Design review of the part shown in the three views and the two pictorial views. Dimensions are in mm from the part's minimum x, y and z. A direction names the side the tool comes from. Give positions to 0.01 mm unless a question says otherwise; leave off trailing zeros. Write each loop counter-clockwise with the first axis right and the second up, starting at its lowest first coordinate (ties: lowest second). Pieces come first, ordered by that corner, then holes. Notation, with made-up numbers: (58, -27.5) -> (90, -27.5) arc R19 cw to (90, 1.5) -> close; hole circle Ø3 at (6, 56). An arc over 180 degrees is marked (long way). Use CSV: the item, a comma, the result in double quotes.
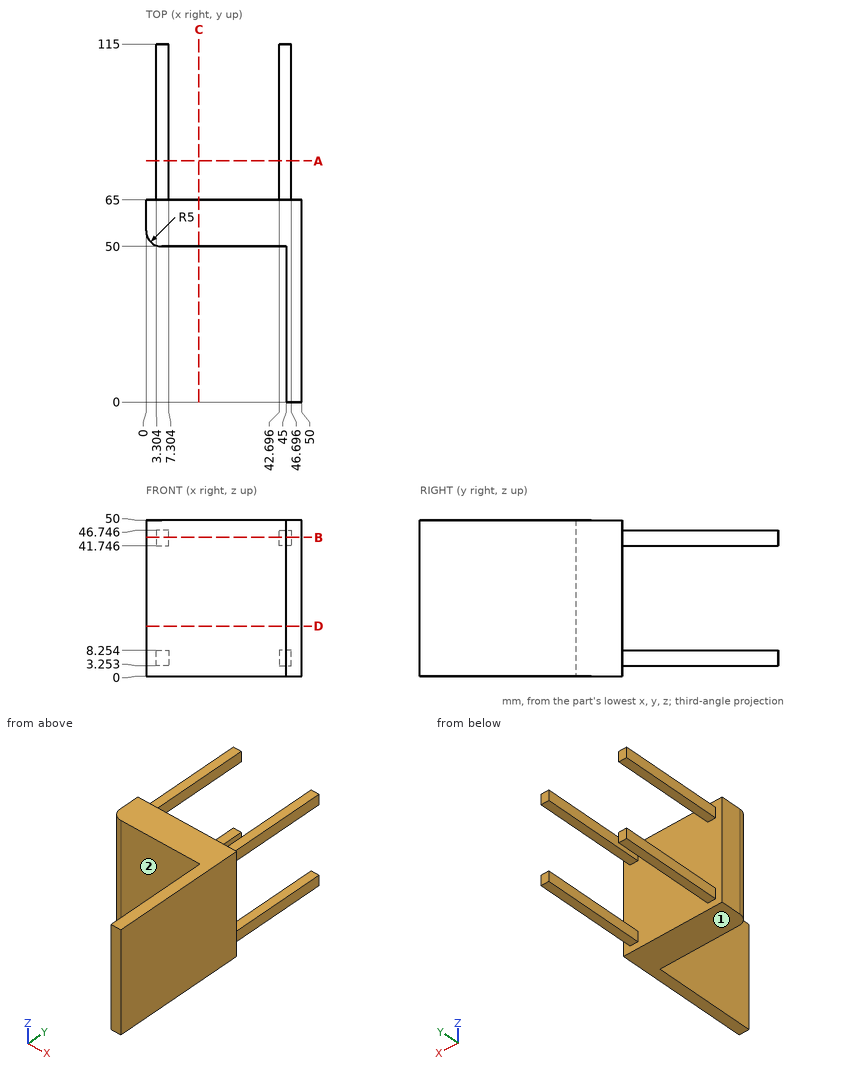
Q1. Consider section B-B (z = 44.5). Write out the cut boundary in (x, y) (1 decimal).
Derived:
outline,"(0, 55) arc R5 ccw to (5, 50) -> (45, 50) -> (45, 0) -> (50, 0) -> (50, 65) -> (46.7, 65) -> (46.7, 115) -> (42.7, 115) -> (42.7, 65) -> (7.3, 65) -> (7.3, 115) -> (3.3, 115) -> (3.3, 65) -> (0, 65) -> close"
Q2. Machinability: for the marked faces 1 and 2, which of the approach directions +Z, -Z, +X, -X, +Y, -Y give a long, thin tool a straight path to every point of the face, cutting with its end or side? Answer none if there is none.
Derived:
face 1,"-Z, +X, -X, +Y, -Y"
face 2,"+Z, -Z, -X, -Y"
Q3. Insertion check: pin 1 (3 mm diameter, centred on x = 40.5, z = 13.5, fed in from -Y); pin 2 (4.5 mm diameter, centred on x = 6, y = 92.5, fed in from +Z); pin 3 (8 mm diameter, centred on x = 27.5, z = 38.5, fed in from +Y). Each pin has a flat end and moves straight along its axis. Give the tip position at first contact, or say it passes through.
Derived:
pin 1,"stops at y = 50"
pin 2,"stops at z = 46.75"
pin 3,"stops at y = 65"
Q4. Consider section D-D (z = 16). Write out the cut boundary in (x, y).
Derived:
outline,"(0, 55) arc R5 ccw to (5, 50) -> (45, 50) -> (45, 0) -> (50, 0) -> (50, 65) -> (0, 65) -> close"
Q5. To check wall thickness, follow probe 1 along Z at (x, y) = (7, 87.5); probe 2 along X at (y, z) = (94, 43.5) (1 decimal); probe 3 along Y at (x, z) = (38, 24.5). State the ranges of each line that lie inside material, in increasing order.
Derived:
probe 1,"z = 3.25 to 8.25, 41.75 to 46.75"
probe 2,"x = 3.3 to 7.3, 42.7 to 46.7"
probe 3,"y = 50 to 65"
Q6. Consider section A-A (y = 77.5). Write out the cut boundary in (x, z) (1 decimal).
Derived:
outline,"(3.3, 3.3) -> (7.3, 3.3) -> (7.3, 8.3) -> (3.3, 8.3) -> close; (3.3, 41.7) -> (7.3, 41.7) -> (7.3, 46.7) -> (3.3, 46.7) -> close; (42.7, 3.3) -> (46.7, 3.3) -> (46.7, 8.3) -> (42.7, 8.3) -> close; (42.7, 41.7) -> (46.7, 41.7) -> (46.7, 46.7) -> (42.7, 46.7) -> close"
Q7. Consider section C-C (x = 17). Write out the cut boundary in (y, z).
Derived:
outline,"(50, 0) -> (65, 0) -> (65, 50) -> (50, 50) -> close"
